Can you work these out from the model? Positions are in its coordinate system, mm. A direction names the side the tool comes from. Give positions to 0.01 mm unless a question says otherwise; leave off trailing zeros. Order: outer loops, then holes, each group sorted by start corner. A loop starts at its lowest first (then second) coordinate and runs counter-clockwise, first axis right, second up. Notation, with made-up numbers: (50.5, 61.25) - (62.5, 61.25) arc R29 cw to (62.5, 88.25) - close; hole circle Ø9 at (-32.75, -16). An arc over 180 degrees is marked (long way). Use one line per item in the form item = value. Start each with the question number.
1) For pin 1 (1.5 mm diameter, centred on x = 29.5, z = 4, fed in from -Y); pin 2 (0.6 mm diameter, centred on y = 35, z = 1.5, fed in from -X); pin 3 (8 mm diameter, centred on x = 10.5, y = 30, fed in from +Z); pin 4 (2 mm diameter, centred on y = 81.5, z = 0.5, fed in from +X), each with a flat end and sliding along its axis, tell me the tip position at first contact or that it passes through.
2) Suppose I cut it at D-D, the plane x = 33.5. Write out the boundary of the cut face in (y, z).
3) Suppose I cut it at C-C, the plane y = 44. Write out the boundary of the cut face in (x, z).
4) Suppose I cut it at A-A, the plane y = 23. Write out the boundary of the cut face in (x, z).
5) We'd pull the mould along X, two halves only. Please class faces 1 (the flat face through (52, 15, 10)), 2 (the flat face through (40, 30, 1)), 3 (the flat face through (10, 30, 1)), 4 (the flat face through (-1, 30, 8)): released by +X, released by -X, zero draft, split by the parting line, or undercut.
6) Please list where these lines run through material, in increasing order: probe 1 along Y at (x, z) = (51.4, 14); probe 2 along Z at (x, y) = (-1, 23); probe 3 along X at (y, z) = (22, 18.75).
7) Suppose I cut it at B-B, the plane z = 14. Write out the boundary of the cut face in (x, y).
8) Which directions (+Z, -Z, +X, -X, +Y, -Y) give clear straight access to the entire face, cutting with the end or side of a thin tool? Please do faces 5 (the flat face through (25, 51, 2)), 6 (the cylindrical face through (-0.99, 29.14, 19.1)), 7 (the flat face through (50, 64, 1)), 8 (the flat face through (25, 100, 1)), 9 (the flat face through (25, 50, 1)).
```python
from build123d import *

# Parameters (mm, degrees)
CYLINDER001_R               = 2
CYLINDER001_DEPTH           = 10
CYLINDER001_PITCH_ANGLE     = 90
CYLINDER001_PLACEMENT_ANGLE = -1e-06
CYLINDER_R                  = 2
CYLINDER_DEPTH              = 10
CYLINDER_PITCH_ANGLE        = 90
CYLINDER_PLACEMENT_ANGLE    = -1e-06
BOX003_W                    = 2
BOX003_H                    = 30
BOX003_DEPTH                = 20
FILLET004_R                 = 3
CYLINDER003_R               = 2
CYLINDER003_DEPTH           = 10
CYLINDER003_PITCH_ANGLE     = 90
CYLINDER003_PLACEMENT_ANGLE = -1e-06
CYLINDER002_R               = 2
CYLINDER002_DEPTH           = 10
CYLINDER002_PITCH_ANGLE     = 90
CYLINDER002_PLACEMENT_ANGLE = -1e-06
BOX004_W                    = 2
BOX004_H                    = 30
BOX004_DEPTH                = 20
FILLET005_R                 = 3
BOX002_W                    = 30
BOX002_H                    = 40
BOX002_DEPTH                = 10
FILLET003_R                 = 1
BOX001_W                    = 30
BOX001_H                    = 20
BOX001_DEPTH                = 10
FILLET002_R                 = 1
BOX_W                       = 50
BOX_H                       = 100
BOX_DEPTH                   = 2
FILLET_R                    = 2
FILLET001_R                 = 2


with BuildPart() as cylinder001:
    # Cylinder001 → Cylinder001 (new body)
    with BuildSketch(Plane.XY):
        Circle(CYLINDER001_R)
    extrude(amount=CYLINDER001_DEPTH)


with BuildPart() as cylinder001_1:
    # Cylinder001 pitch: moved
    add(cylinder001.part.rotate(Axis((0, 0, 0), (0, 1, 0)), CYLINDER001_PITCH_ANGLE))


with BuildPart() as cylinder001_2:
    # Cylinder001 placement: moved
    add(cylinder001_1.part.moved(Location((-6, 23, 14))).rotate(Axis((-6, 23, 14), (0, 0, 1)), CYLINDER001_PLACEMENT_ANGLE))


with BuildPart() as cylinder:
    # Cylinder → Cylinder (new body)
    with BuildSketch(Plane.XY):
        Circle(CYLINDER_R)
    extrude(amount=CYLINDER_DEPTH)


with BuildPart() as cylinder_1:
    # Cylinder pitch: moved
    add(cylinder.part.rotate(Axis((0, 0, 0), (0, 1, 0)), CYLINDER_PITCH_ANGLE))


with BuildPart() as cylinder_2:
    # Cylinder placement: moved
    add(cylinder_1.part.moved(Location((-6, 7, 14))).rotate(Axis((-6, 7, 14), (0, 0, 1)), CYLINDER_PLACEMENT_ANGLE))


with BuildPart() as cut003:
    # Box003 → Box003 (new body)
    with BuildSketch(Plane(origin=(-2, 0, 0), x_dir=(1, 0, 0), z_dir=(0, 0, 1))):
        with Locations((1, 15)):
            Rectangle(BOX003_W, BOX003_H)
    extrude(amount=BOX003_DEPTH)

    # Fillet004
    fillet004_edges = [cut003.edges().sort_by_distance(p)[0] for p in [
        (-1, 0, 20),
        (-1, 30, 20),
    ]]
    fillet(fillet004_edges, radius=FILLET004_R)

    # Cut002: cut Cylinder
    add(cylinder_2.part, mode=Mode.SUBTRACT)

    # Cut003: cut Cylinder001
    add(cylinder001_2.part, mode=Mode.SUBTRACT)


with BuildPart() as cylinder003:
    # Cylinder003 → Cylinder003 (new body)
    with BuildSketch(Plane.XY):
        Circle(CYLINDER003_R)
    extrude(amount=CYLINDER003_DEPTH)


with BuildPart() as cylinder003_1:
    # Cylinder003 pitch: moved
    add(cylinder003.part.rotate(Axis((0, 0, 0), (0, 1, 0)), CYLINDER003_PITCH_ANGLE))


with BuildPart() as cylinder003_2:
    # Cylinder003 placement: moved
    add(cylinder003_1.part.moved(Location((-6, 23, 14))).rotate(Axis((-6, 23, 14), (0, 0, 1)), CYLINDER003_PLACEMENT_ANGLE))


with BuildPart() as cylinder002:
    # Cylinder002 → Cylinder002 (new body)
    with BuildSketch(Plane.XY):
        Circle(CYLINDER002_R)
    extrude(amount=CYLINDER002_DEPTH)


with BuildPart() as cylinder002_1:
    # Cylinder002 pitch: moved
    add(cylinder002.part.rotate(Axis((0, 0, 0), (0, 1, 0)), CYLINDER002_PITCH_ANGLE))


with BuildPart() as cylinder002_2:
    # Cylinder002 placement: moved
    add(cylinder002_1.part.moved(Location((-6, 7, 14))).rotate(Axis((-6, 7, 14), (0, 0, 1)), CYLINDER002_PLACEMENT_ANGLE))


with BuildPart() as cut005:
    # Box004 → Box004 (new body)
    with BuildSketch(Plane(origin=(-2, 0, 0), x_dir=(1, 0, 0), z_dir=(0, 0, 1))):
        with Locations((1, 15)):
            Rectangle(BOX004_W, BOX004_H)
    extrude(amount=BOX004_DEPTH)

    # Fillet005
    fillet005_edges = [cut005.edges().sort_by_distance(p)[0] for p in [
        (-1, 0, 20),
        (-1, 30, 20),
    ]]
    fillet(fillet005_edges, radius=FILLET005_R)

    # Cut004: cut Cylinder002
    add(cylinder002_2.part, mode=Mode.SUBTRACT)

    # Cut005: cut Cylinder003
    add(cylinder003_2.part, mode=Mode.SUBTRACT)


with BuildPart() as cut005_1:
    # Cut005 placement: moved
    add(cut005.part.moved(Location((52, 0, 0))))


with BuildPart() as fillet003:
    # Box002 → Box002 (new body)
    with BuildSketch(Plane(origin=(10, 10, 0), x_dir=(1, 0, 0), z_dir=(0, 0, 1))):
        with Locations((15, 20)):
            Rectangle(BOX002_W, BOX002_H)
    extrude(amount=BOX002_DEPTH)

    # Fillet003
    fillet003_edges = [fillet003.edges().sort_by_distance(p)[0] for p in [
        (10, 10, 5),
        (10, 50, 5),
        (40, 10, 5),
        (40, 50, 5),
    ]]
    fillet(fillet003_edges, radius=FILLET003_R)


with BuildPart() as fillet002:
    # Box001 → Box001 (new body)
    with BuildSketch(Plane(origin=(10, 70, 0), x_dir=(1, 0, 0), z_dir=(0, 0, 1))):
        with Locations((15, 10)):
            Rectangle(BOX001_W, BOX001_H)
    extrude(amount=BOX001_DEPTH)

    # Fillet002
    fillet002_edges = [fillet002.edges().sort_by_distance(p)[0] for p in [
        (10, 70, 5),
        (10, 90, 5),
        (40, 70, 5),
        (40, 90, 5),
    ]]
    fillet(fillet002_edges, radius=FILLET002_R)


with BuildPart() as fusion:
    # Box → Box (new body)
    with BuildSketch(Plane.XY):
        with Locations((25, 50)):
            Rectangle(BOX_W, BOX_H)
    extrude(amount=BOX_DEPTH)

    # Fillet
    fillet_edges = [fusion.edges().sort_by_distance(p)[0] for p in [
        (50, 100, 1),
    ]]
    fillet(fillet_edges, radius=FILLET_R)

    # Fillet001
    fillet001_edges = [fusion.edges().sort_by_distance(p)[0] for p in [
        (0, 100, 1),
    ]]
    fillet(fillet001_edges, radius=FILLET001_R)

    # Cut: cut Fillet002
    add(fillet002.part, mode=Mode.SUBTRACT)

    # Cut001: cut Fillet003
    add(fillet003.part, mode=Mode.SUBTRACT)

    # Fusion: union Cut003, Cut005
    add(cut003.part)
    add(cut005_1.part)


solid = fusion.part
```
Result sheet:
q1.pin_1 = through
q1.pin_2 = 0
q1.pin_3 = 2
q1.pin_4 = 50
q2.outline = (0, 0) - (10, 0) - (10, 2) - (0, 2) - close; (50, 0) - (70, 0) - (70, 2) - (50, 2) - close; (90, 0) - (100, 0) - (100, 2) - (90, 2) - close
q3.outline = (0, 0) - (10, 0) - (10, 2) - (0, 2) - close; (40, 0) - (50, 0) - (50, 2) - (40, 2) - close
q4.outline = (-2, 0) - (10, 0) - (10, 2) - (0, 2) - (0, 12) - (-2, 12) - close; (-2, 16) - (0, 16) - (0, 20) - (-2, 20) - close; (40, 0) - (52, 0) - (52, 12) - (50, 12) - (50, 2) - (40, 2) - close; (50, 16) - (52, 16) - (52, 20) - (50, 20) - close
q5.face_1 = released by +X
q5.face_2 = undercut
q5.face_3 = undercut
q5.face_4 = zero draft
q6.probe_1 = 0 to 5, 9 to 21, 25 to 30
q6.probe_2 = 0 to 12, 16 to 20
q6.probe_3 = -2 to 0, 50 to 52
q7.outline = (-2, 0) - (0, 0) - (0, 5) - (-2, 5) - close; (-2, 9) - (0, 9) - (0, 21) - (-2, 21) - close; (-2, 25) - (0, 25) - (0, 30) - (-2, 30) - close; (50, 0) - (52, 0) - (52, 5) - (50, 5) - close; (50, 9) - (52, 9) - (52, 21) - (50, 21) - close; (50, 25) - (52, 25) - (52, 30) - (50, 30) - close
q8.face_5 = +Z, +Y, -Y
q8.face_6 = +Z, +X, -X, +Y
q8.face_7 = +Z, -Z, +X, +Y
q8.face_8 = +Z, -Z, +X, -X, +Y
q8.face_9 = +Z, -Z
